Job drawing, mm, ordinate dimensions from the low corner. One solid piece. A direction names the side the tool comes from. Coordinates: 2 decimals unless noted, no trailing zeros. Order: outer loops, then holes, each group sorted by start corner. A loop starts at its lowest first (then second) coordinate and runs counter-clockwise, first axis right, second up. Notation, with made-up numbers: M 21,21.25 L 80,21.25 A22 ccw 80,33.25 Z; hole C 45.25,80.25 d1. An arc over 180 degrees is marked long. Write item = value, one per line.
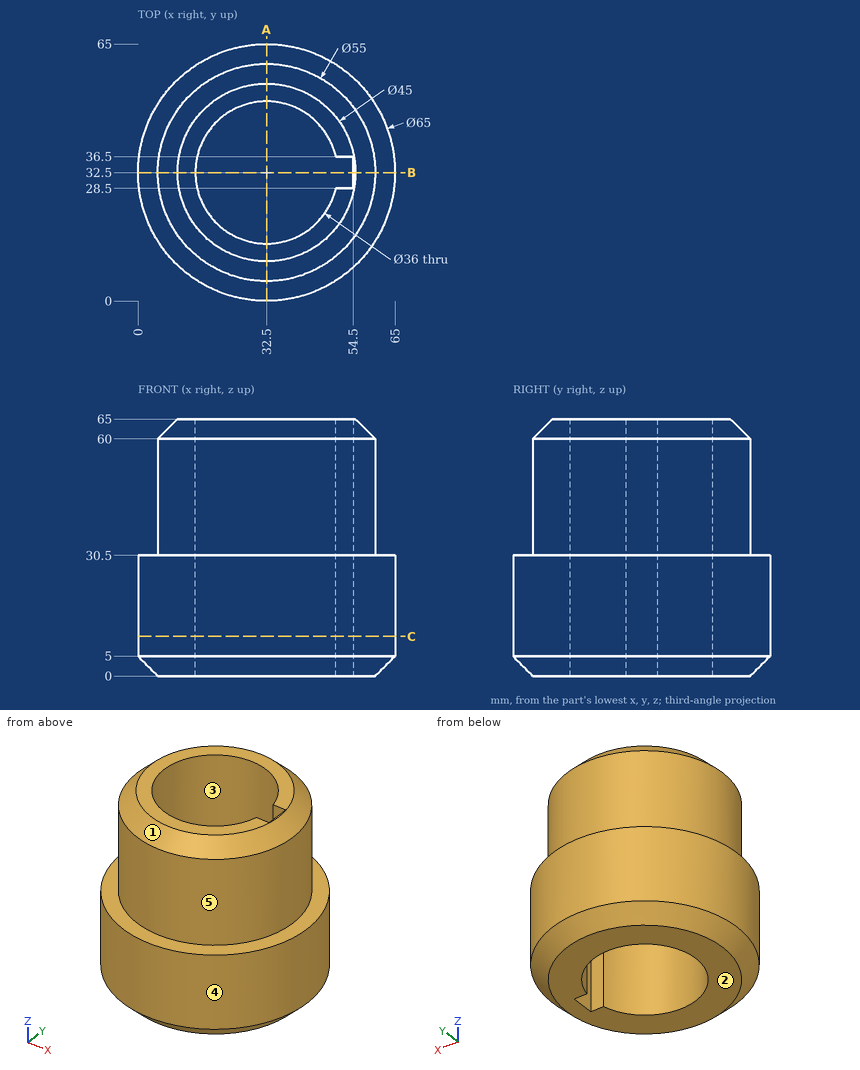
(1) Tool access for the marked faces 4 and 5: list every direction of +Z, -Z, +X, -X, +Y, -Y with a clear straight run to the whole face (end or side of a thin tool).
Evaluation:
face_4 = +Z, -Z
face_5 = +Z
(2) Wall check: line 1 (X direction, y = 32, z = 19); line 2 (Y direction, x = 32, z = 14); line 3 (X direction, y = 32, z = 50). Give the ranges that are in metal, low to high. Write a range as from..to.
Evaluation:
line_1 = 0..14.51, 54.5..65
line_2 = 0..14.51, 50.49..65
line_3 = 5..14.51, 54.5..60
(3) Slice it at B-B, the plane y = 32.5. Write the cut outline in (x, z), then the cut area to 3 significant figures.
Evaluation:
outline = M 0,5 L 5,0 L 14.5,0 L 14.5,65 L 10,65 L 5,60 L 5,30.5 L 0,30.5 Z; M 54.5,0 L 60,0 L 65,5 L 65,30.5 L 60,30.5 L 60,60 L 55,65 L 54.5,65 Z
area = 1,230 mm²
(4) Slice it at A-A, the plane x = 32.5. Write the cut outline in (y, z).
Evaluation:
outline = M 0,5 L 5,0 L 14.5,0 L 14.5,65 L 10,65 L 5,60 L 5,30.5 L 0,30.5 Z; M 50.5,0 L 60,0 L 65,5 L 65,30.5 L 60,30.5 L 60,60 L 55,65 L 50.5,65 Z
(5) Pin check, flat tips, straight feed: pin 1 Ø3.5 at (x, z) = (51.5, 23.5) entering from -Y; pin 2 Ø8 at (x, z) = (7, 8.5) entering from +Y; pin 3 Ø1.3 at (x, z) = (51.5, 17.5) entering from +Y; pin 4 Ø2 at (x, y) = (58, 9) entering from +Z. Stop position of each tip, or through.
Evaluation:
pin_1 = 4.96
pin_2 = 56.87
pin_3 = 59.32
pin_4 = through
(6) Pull direction X, two halves, no side cores. Call the marked faces 1, 2 and 3: +X half, -X half, draft (parallel to the pull), parting line (faces both ways), or undercut.
Evaluation:
face_1 = parting line
face_2 = draft
face_3 = undercut
(7) Slice it at C-C, the plane z = 10. Write the cut outline in (x, y).
Evaluation:
outline = C 32.5,32.5 d65; hole M 50.05,28.5 L 54.5,28.5 L 54.5,36.5 L 50.05,36.5 A18 ccw long Z
